from build123d import *

# Parameters (mm, degrees)
SKETCH_1_R      = 1.5
EXTRUDE_3_DEPTH = 4
SKETCH_1_8_W    = 25
SKETCH_1_8_H    = 150
EXTRUDE_4_DEPTH = 4
FILLET_1_R      = 3


with BuildPart() as part:
    # Sketch 1 → Extrude 3 (new body)
    with BuildSketch(Plane(origin=(0, 0, 0), x_dir=(1, 0, 0), z_dir=(0, 1, 0))):
        with BuildLine():
            Line((97.132652086, -142.242252719), (105.132652086, -142.242252719))
            Line((105.132652086, -142.242252719), (105.132652086, -127.242252719))
            ThreePointArc((105.132652086, -127.242252719), (106.632652086, -125.742252719), (108.132652086, -127.242252719))
            Line((108.132652086, -127.242252719), (108.132652086, -142.242252719))
            Line((108.132652086, -142.242252719), (113.132652086, -142.242252719))
            Line((113.132652086, -142.242252719), (113.132652086, -127.242252719))
            ThreePointArc((113.132652086, -127.242252719), (114.632652086, -125.742252719), (116.132652086, -127.242252719))
            Line((116.132652086, -127.242252719), (116.132652086, -142.242252719))
            Line((116.132652086, -142.242252719), (158.517652086, -142.242252719))
            Line((158.517652086, -142.242252719), (158.517652086, 7.757747281))
            Line((158.517652086, 7.757747281), (0.517652086, 7.757747281))
            Line((0.517652086, 7.757747281), (0.517652086, -95.742252719))
            ThreePointArc((0.517652086, -95.742252719), (1.578312257, -96.181592547), (2.017652086, -97.242252719))
            Line((2.017652086, -97.242252719), (2.017652086, -102.242252719))
            Line((2.017652086, -102.242252719), (7.017652086, -102.242252719))
            Line((7.017652086, -102.242252719), (7.017652086, -97.242252719))
            ThreePointArc((7.017652086, -97.242252719), (8.517652086, -95.742252719), (10.017652086, -97.242252719))
            Line((10.017652086, -97.242252719), (10.017652086, -102.242252719))
            Line((10.017652086, -102.242252719), (15.017652086, -102.242252719))
            Line((15.017652086, -102.242252719), (15.017652086, -97.242252719))
            ThreePointArc((15.017652086, -97.242252719), (16.517652086, -95.742252719), (18.017652086, -97.242252719))
            Line((18.017652086, -97.242252719), (18.017652086, -102.242252719))
            Line((18.017652086, -102.242252719), (23.017652086, -102.242252719))
            Line((23.017652086, -102.242252719), (23.017652086, -97.242252719))
            ThreePointArc((23.017652086, -97.242252719), (24.517652086, -95.742252719), (26.017652086, -97.242252719))
            Line((26.017652086, -97.242252719), (26.017652086, -102.242252719))
            Line((26.017652086, -102.242252719), (31.017652086, -102.242252719))
            Line((31.017652086, -102.242252719), (31.017652086, -97.242252719))
            ThreePointArc((31.017652086, -97.242252719), (32.517652086, -95.742252719), (34.017652086, -97.242252719))
            Line((34.017652086, -97.242252719), (34.017652086, -102.242252719))
            Line((34.017652086, -102.242252719), (39.017652086, -102.242252719))
            Line((39.017652086, -102.242252719), (39.017652086, -97.242252719))
            ThreePointArc((39.017652086, -97.242252719), (40.517652086, -95.742252719), (42.017652086, -97.242252719))
            Line((42.017652086, -97.242252719), (42.017652086, -102.242252719))
            Line((42.017652086, -102.242252719), (47.132652086, -102.242252719))
            Line((47.132652086, -102.242252719), (47.132652086, -32.242252719))
            Line((47.132652086, -32.242252719), (122.132652086, -32.242252719))
            Line((122.132652086, -32.242252719), (122.132652086, -87.242252719))
            Line((122.132652086, -87.242252719), (97.132652086, -87.242252719))
            Line((97.132652086, -87.242252719), (97.132652086, -142.242252719))
        make_face()
        with Locations(Location((101.932652086, -117.242252719, 0), (0, 0, 270))):
            Circle(SKETCH_1_R, mode=Mode.SUBTRACT)
        with Locations(Location((119.632652086, -117.242252719, 0), (0, 0, 270))):
            Circle(SKETCH_1_R, mode=Mode.SUBTRACT)
        with Locations(Location((105.422652086, -92.242252719, 0), (0, 0, 270))):
            Circle(SKETCH_1_R, mode=Mode.SUBTRACT)
        with Locations(Location((100.132652086, -110.242252719, 0), (0, 0, 270))):
            Circle(SKETCH_1_R, mode=Mode.SUBTRACT)
        with Locations(Location((105.132652086, -23.242252719, 0), (0, 0, 270))):
            Circle(SKETCH_1_R, mode=Mode.SUBTRACT)
        with Locations(Location((41.132652086, -79.242252719, 0), (0, 0, 270))):
            Circle(SKETCH_1_R, mode=Mode.SUBTRACT)
        with Locations(Location((143.517652086, -100.242252719, 0), (0, 0, 270))):
            Circle(SKETCH_1_R, mode=Mode.SUBTRACT)
        with Locations(Location((154.017652086, -89.742252719, 0), (0, 0, 270))):
            Circle(SKETCH_1_R, mode=Mode.SUBTRACT)
        with Locations(Location((143.517652086, -79.242252719, 0), (0, 0, 270))):
            Circle(SKETCH_1_R, mode=Mode.SUBTRACT)
        with Locations(Location((41.132652086, -39.242252719, 0), (0, 0, 270))):
            Circle(SKETCH_1_R, mode=Mode.SUBTRACT)
        with Locations(Location((64.132652086, -23.242252719, 0), (0, 0, 270))):
            Circle(SKETCH_1_R, mode=Mode.SUBTRACT)
    extrude(amount=EXTRUDE_3_DEPTH)

    # Sketch 1_8 → Extrude 4 (add)
    with BuildSketch(Plane(origin=(0, 0, 0), x_dir=(1, 0, 0), z_dir=(0, 1, 0))):
        with Locations((171.017652086, -67.242252719)):
            Rectangle(SKETCH_1_8_W, SKETCH_1_8_H)
    extrude(amount=EXTRUDE_4_DEPTH)

    # Fillet 1
    fillet_1_edges = [part.edges().sort_by_distance(p)[0] for p in [
        (183.517652086, 2, 142.242252719),
        (183.517652086, 2, -7.757747281),
        (0.517652086, 2, -7.757747281),
        (97.132652086, 2, 87.242252719),
        (122.132652086, 2, 87.242252719),
        (122.132652086, 2, 32.242252719),
        (47.132652086, 2, 32.242252719),
        (47.132652086, 2, 102.242252719),
    ]]
    fillet(fillet_1_edges, radius=FILLET_1_R)


solid = part.part
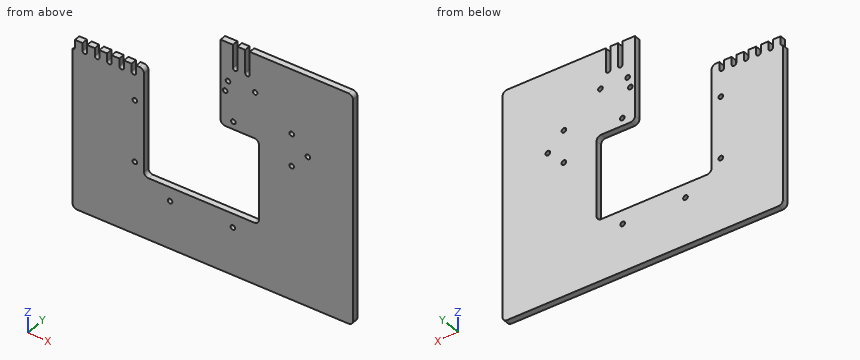
Input: part model. Units: mm. Frame: model coordinates. Coordinates: 2 decimals unless noted, no trailing zeros. Loops run counter-clockwise (first coordinate to the right, second up) from the corner with the lowest first, then second, coordinate; pieces in that order, holes last.
Q1. Contact query for flat-ended pins moving along their axis: pin 1 (2.5 mm diameter, centred on x = 143.52, z = 100.24, fed in from +Y); pin 2 (1.2 mm diameter, centred on y = 2, z = 100, fed in from -X); pin 3 (1.2 mm diameter, centred on x = 13.5, y = 1.5, fed in from +Z). Output: stop coordinate, or through.
Q2. Cut plane C-C (x = 56). Output: boundary loops of the cut face in (y, z).
Q3. Cut plane D-D (y = 2.1). Give the number of separate pieces and of enclosed holes in the cut face, then the cut area to 3 significant figures.
Q4. Cut plane B-B (z = 58). Output: boundary loops of the cut face in (x, y).
Q5. Cut plane A-A (z = 131.5). Output: boundary loops of the cut face in (x, y).
Q6. Material intervals for line 1 (X direction, y = 2.05, z = 132.5); line 2 (Z direction, x = 119.5, y = 3.5); line 3 (X direction, y = 3, z = 79), sorted ascending.
Working result:
1. pin 1: passes through
1. pin 2: stops at x = 2.02
1. pin 3: stops at z = 102.24
2. outline: (0, -7.76) - (4, -7.76) - (4, 32.24) - (0, 32.24) - close
3. separate pieces: 1
3. enclosed holes: 11
3. area: 18,400 mm2
4. outline: (0.52, 0) - (47.13, 0) - (47.13, 4) - (0.52, 4) - close; (122.13, 0) - (183.52, 0) - (183.52, 4) - (122.13, 4) - close
5. outline: (97.13, 0) - (105.13, 0) - (105.13, 4) - (97.13, 4) - close; (108.13, 0) - (113.13, 0) - (113.13, 4) - (108.13, 4) - close; (116.13, 0) - (183.52, 0) - (183.52, 4) - (116.13, 4) - close
6. line 1: x = 97.13 to 105.13, 108.13 to 113.13, 116.13 to 183.52
6. line 2: z = -7.76 to 32.26, 87.22 to 115.75, 118.74 to 142.24
6. line 3: x = 0.52 to 39.65, 42.61 to 47.13, 122.13 to 142.04, 145 to 183.52
